Source: CAD feature listing. Evaluate the final solid. Frame: model axes, mm. Face numbers are marked on the shaded views. A direction names the side the tool comes from. Round coordinates to 2 decimals unless told otherwise and drop trailing zeros. Loops run counter-clockwise (first coordinate to the right, second up) from the corner with the lowest first, then second, coordinate; pieces in that order, holes last. Notation, with made-up numbers: M 63.25,70.25 L 80.25,70.25 A11 ccw 80.25,84.25 Z; hole C 87,15.5 d1. An arc over 180 degrees is marked long. Write each question's results on one line, items separated by ' | '. Start each with the question number.
1. Ray query, line 1 (Y direction, x = 28.8, z = 10.75); line 2 (Z direction, x = 5.25, y = -5.7); line 3 (Y direction, x = 10.5, z = 5.5). Return the intervals inside material, ascending.
2. Section B-B on y = -5.7. Output: boundary loops of the cut face in (x, z).
3. Contact query for flat-ended pins moving along their axis: pin 1 Ø5 at (x, z) = (4, 7.5) entering from -Y; pin 2 Ø2 at (y, z) = (-5.7, 2.2) entering from -X; pin 3 Ø5 at (y, z) = (-4, 5) entering from +X. Output: stop coordinate, or through.
4. Section C-C on x = 8.5. Output: boundary loops of the cut face in (y, z).
5. Set-up query: the marked faces 1, 2 and 3. Return all of +Z, -Z, +X, -X, +Y, -Y with unobstructed straight access to the full face (end or side cutting, diameter ignored); none if empty.
6. Draft query along X for the marked faces 4, 5 and 6. Return one class per face: released by +X, released by -X, zero draft, split by the parting line, or undercut.
7. Section A-A on x = 28.8. Output: boundary loops of the cut face in (y, z).
8. Section D-D on y = -8.5. Output: boundary loops of the cut face in (x, z), and give its area (4 significant figures).
from build123d import *

# Parameters (mm, degrees)
CROQUIS1_W              = 18
CROQUIS1_H              = 11
SALIENTE_EXTRUIR1_DEPTH = 6
CROQUIS3_W              = 12
CROQUIS3_H              = 11.002490455
SALIENTE_EXTRUIR2_DEPTH = 8
CROQUIS4_W              = 3
CROQUIS4_H              = 11.002490455
SALIENTE_EXTRUIR3_DEPTH = 6
CROQUIS5_R              = 1.25
CORTAR_EXTRUIR1_DEPTH   = 10
CROQUIS6_R              = 1.25
CORTAR_EXTRUIR2_DEPTH   = 10
CHAFL_N1_SIZE           = 10
CHAFL_N2_SIZE           = 6
REDONDEO1_R             = 2


with BuildPart() as part:
    # Croquis1 → Saliente-Extruir1 (new body)
    with BuildSketch(Plane.XY):
        with Locations((9, -5.5)):
            Rectangle(CROQUIS1_W, CROQUIS1_H)
    extrude(amount=SALIENTE_EXTRUIR1_DEPTH)

    # Croquis3 → Saliente-Extruir2 (add)
    with BuildSketch(Plane(origin=(18, 0, 0), x_dir=(0, 0, -1), z_dir=(1, 0, 0))):
        with Locations((-6, -5.501245228)):
            Rectangle(CROQUIS3_W, CROQUIS3_H)
    extrude(amount=SALIENTE_EXTRUIR2_DEPTH)

    # Croquis4 → Saliente-Extruir3 (add)
    with BuildSketch(Plane(origin=(26, 0, 0), x_dir=(0, 0, -1), z_dir=(1, 0, 0))):
        with Locations((-10.5, -5.501245228)):
            Rectangle(CROQUIS4_W, CROQUIS4_H)
    extrude(amount=SALIENTE_EXTRUIR3_DEPTH)

    # Croquis5 → Cortar-Extruir1 (cut)
    with BuildSketch(Plane.ZY):
        with Locations(Location((2.2, -5.7, 0), (0, 0, 270))):
            Circle(CROQUIS5_R)
    extrude(amount=-CORTAR_EXTRUIR1_DEPTH, mode=Mode.SUBTRACT)

    # Croquis6 → Cortar-Extruir2 (cut)
    with BuildSketch(Plane.XY.offset(12)):
        with Locations((28.8, -6.002490455)):
            Circle(CROQUIS6_R)
    extrude(amount=-CORTAR_EXTRUIR2_DEPTH, mode=Mode.SUBTRACT)

    # Chaflán1
    # the kernel refuses this chamfer: 10 mm, written as the material it takes off along each edge
    with BuildSketch(Plane(origin=(26, -36.719320335, 0), x_dir=(0, 0, 1), z_dir=(0, 1, 0))) as chafl_n1_piece_1_section:
        Polygon((CHAFL_N1_SIZE, 0), (0, -CHAFL_N1_SIZE), (0, 0), align=None)
    chafl_n1_piece_1 = extrude(amount=62.436150214, mode=Mode.PRIVATE)
    chafl_n1_piece_1 = split(chafl_n1_piece_1, bisect_by=Plane(origin=(26, -36.719320335, 9), z_dir=(0, 0, -1)), keep=Keep.TOP, mode=Mode.PRIVATE)
    add(chafl_n1_piece_1, mode=Mode.SUBTRACT)

    # Chaflán2
    chafl_n2_edges = [part.edges().sort_by_distance(p)[0] for p in [
        (18, -5.501245227, 12),
    ]]
    chamfer(chafl_n2_edges, length=CHAFL_N2_SIZE)

    # Redondeo1
    redondeo1_edges = [part.edges().sort_by_distance(p)[0] for p in [
        (18, -5.5, 6),
        (16, -5.5, 0),
        (25, -5.501245227, 9),
        (24, -5.501245227, 12),
    ]]
    fillet(redondeo1_edges, radius=REDONDEO1_R)


solid = part.part
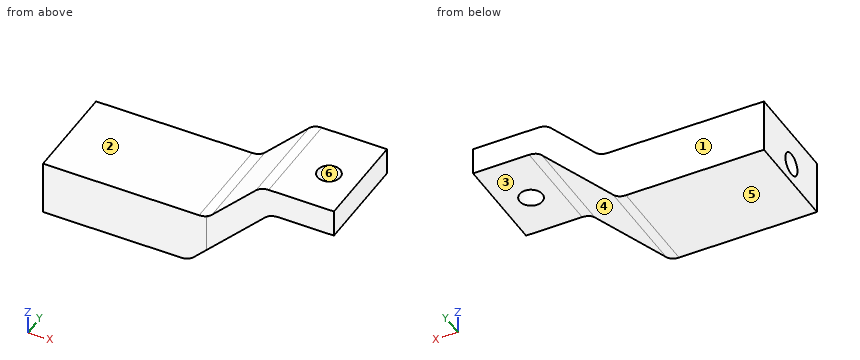
Taken from the geometry:
1) line 1: -11 to -7.25, -4.75 to 0 | line 2: 0 to 0.95, 3.45 to 6 | line 3: -11 to 0
2) outline: M 0,0 L 15.17,0 A2 ccw 16.59,0.59 L 24.41,8.41 A2 cw 25.83,9 L 27.59,9 L 27.59,12 L 24.83,12 A2 ccw 23.41,11.41 L 18.59,6.59 A2 cw 17.17,6 L 0,6 L 0,3.45 L 10,3.45 L 10,0.95 L 0,0.95 Z; M 30.01,9 L 32,9 L 32,12 L 30.01,12 Z
3) pin 1: y = -11 | pin 2: x = 10 | pin 3: x = 23.5
4) outline: M -11,0 L 0,0 L 0,6 L -11,6 Z; hole C -5.7,2.2 d2.5
5) face 1: +Z, -Z, +X, -X, +Y | face 2: +Z, -X, +Y, -Y | face 3: -Z, +X, +Y, -Y
6) face 4: released by +X | face 5: zero draft | face 6: undercut
7) outline: M -11,9 L -7.25,9 L -7.25,12 L -11,12 Z; M -4.75,9 L 0,9 L 0,12 L -4.75,12 Z
8) outline: M 0,0 L 15.17,0 A2 ccw 16.59,0.59 L 24.41,8.41 A2 cw 25.83,9 L 32,9 L 32,12 L 24.83,12 A2 ccw 23.41,11.41 L 18.59,6.59 A2 cw 17.17,6 L 0,6 Z | area: 154.5 mm^2
